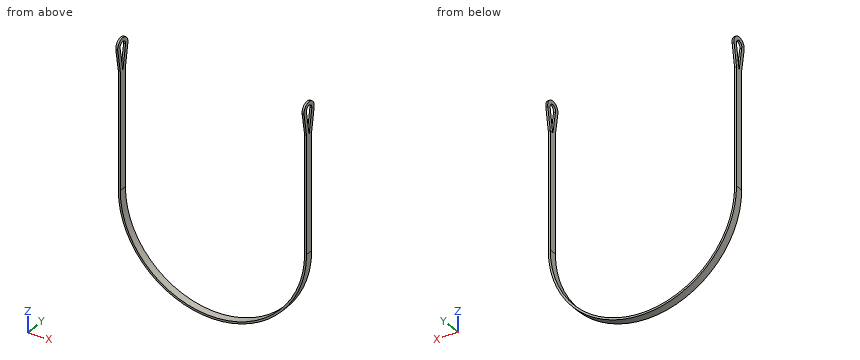
from build123d import *

# Parameters (mm, degrees)
F1_W = 12.7
F1_H = 50.8
F5_W = 12.7
F5_H = 23.8677083557


with BuildPart() as f2:
    # F2: sweep along a path in F0
    with BuildLine(Plane.XZ) as f2_path:
        Line((-609.6, 0), (-609.6, -762))
        ThreePointArc((-609.6, -762), (0, -1371.6), (609.6, -762))
        Line((609.6, -762), (609.6, 0))
    # F1 (on Top) → F2 (sweep)
    with BuildSketch(Plane.XY):
        with Locations((-609.6, 0)):
            Rectangle(F1_W, F1_H)
    sweep(path=f2_path.line)

    # F6: sweep along a path in F4
    with BuildLine(Plane.YZ.offset(609.6)) as f6_path:
        Line((-12.7, 0), (-37.5594649148, 146.0049554096))
        ThreePointArc((-37.5594649148, 146.0049554096), (0, 190.5), (37.5594649148, 146.0049554096))
        Line((37.5594649148, 146.0049554096), (12.7, 0))
    # F5 (on face) → F6 (sweep)
    with BuildSketch(Plane.XY):
        with Locations((609.6, -13.4661458221)):
            Rectangle(F5_W, F5_H)
    sweep(path=f6_path.line)

    # F7: F2 across plane


with BuildPart() as f2_1:
    add(f2.part)
    add(f2.part.mirror(Plane.YZ))


solid = f2_1.part
Input: part model. Units: mm. Frame: model coordinates. Coordinates: 2 decimals unless noted, no trailing zeros. Order: outer loops, then holes, each group sorted by start corner. A loop starts at its lowest first (then second) coordinate and runs counter-clockwise, first axis right, second up. Notation, with made-up numbers: M 88,-18 L 128,-18 A15 ccw 128,8 Z; hole C -39.5,87.25 d4. An arc over 180 degrees is marked long. Answer as CSV lines item,"result".
1. Section B-B (x = 0). Return the cut outline in (y, z).
Reported:
outline,"M -25.4,-1377.95 L 25.4,-1377.95 L 25.4,-1365.25 L -25.4,-1365.25 Z"
2. Section C-C (z = -802). Return the cut outline in (x, y), then the cut area to 3 significant figures.
Reported:
outline,"M -614.65,-25.4 L -601.92,-25.4 L -601.92,25.4 L -614.65,25.4 Z; M 601.92,-25.4 L 614.65,-25.4 L 614.65,25.4 L 601.92,25.4 Z"
area,"1,290 mm2"
3. Material intervals for line 1 (Y direction, x = -611.5, z = 152.4); line 2 (Y direction, x = 608, z = 152); line 3 (X direction, y = 0, z = -146), sorted ascending. Write a range as from..to.
Reported:
line 1,"-50.66..-27.16, 27.16..50.66"
line 2,"-50.66..-27.15, 27.15..50.66"
line 3,"-615.95..-603.25, 603.25..615.95"
4. Section A-A (z = -384.5). Return the cut outline in (x, y), then the cut area to 3 significant figures.
Reported:
outline,"M -615.95,-25.4 L -603.25,-25.4 L -603.25,25.4 L -615.95,25.4 Z; M 603.25,-25.4 L 615.95,-25.4 L 615.95,25.4 L 603.25,25.4 Z"
area,"1,290 mm2"
5. First-contact query: P1, Ø6.5, axis at x = -607, y = 7.5, coming from the +Z side; P2, Ø4, axis at x = 606.5, y = 2, coming from the +Z side; P3, Ø8, axis at x = -290.5, y = 21.5, coming from the +Z side. Flat tips, straight axial feed; report the tip coordinate or a pass-through.
Reported:
P1,"z = 202.89"
P2,"z = 203.06"
P3,"z = -1288.48"
6. Section D-D (x = -478). Return the cut outline in (y, z), then the cut area to 3 significant figures.
Reported:
outline,"M -25.4,-1150.47 L 25.4,-1150.47 L 25.4,-1130 L -25.4,-1130 Z"
area,"1,040 mm2"
